Autodesk Inventor part; units mm, degrees
ref_plane "YZ Plane" through (0, 0, 0) normal (1, 0, 0) x (0, 1, 0)
ref_plane "XZ Plane" through (0, 0, 0) normal (0, 1, 0) x (-1, 0, 0)
ref_plane "XY Plane" through (0, 0, 0) normal (0, 0, 1) x (1, 0, 0)
sketch "Sketch1" plane through (0, 0, 0) normal (0, 0, 1) x (1, 0, 0)
  line L0 (0, 0) -> (27.9, 0)
  line L1 (27.9, 0) -> (27.9, -22.1)
  line L2 (27.9, -22.1) -> (0, -22.1)
  line L3 (0, -22.1) -> (0, 0)
  dimension "d0" = 27.9
  dimension "d1" = 22.1
extrude "Extrusion1" add sketch "Sketch1" along normal blind 2.5
sketch "Sketch2" plane through (0, 0, 0) normal (0, 1, 0) x (1, 0, 0)
  line L0 (1.95, -4.5) -> (25.95, -4.5) construction
  line L1 (4.95, -7.5) -> (22.95, -7.5)
  line L2 (22.95, -1.5) -> (4.95, -1.5)
  arc A0 (4.95, -1.5) -> (4.95, -7.5) centre (4.95, -4.5) ccw
  arc A1 (22.95, -7.5) -> (22.95, -1.5) centre (22.95, -4.5) ccw
  line L3 (27.9, 0) -> (27.9, -2.5)
  line L4 (0, 0) -> (0, -2.5)
  line L5 (27.9, -2.5) -> (0, -2.5)
  circle A2 centre (5.95, -4.5) radius 1.6
  circle A3 centre (21.95, -4.5) radius 1.6
  line L6 (4.752, -3.4394) -> (4.752, -5.5606)
  line L7 (0, 0) -> (27.9, 0)
  line L8 (13.95, 0) -> (13.95, -7.0714)
  point P0 (13.95, -4.5)
  dimension "d4" = 6
  dimension "d5" = 24
  dimension "d8" = 1
  dimension "d9" = 3.2
  dimension "d10" = 3.2
  dimension "d11" = 16
  dimension "d12" = 8
extrude "Extrusion2" add sketch "Sketch2" along normal blind 1.5 contours A0 L5 A1 L1 | A0 L2 L8 L5 | L5 L8 L2 A1
fillet "Fillet1" radius 0.3 4 edges at (1.95, 1.5, 4.5) (13.95, 1.5, 7.5) (25.95, 1.5, 4.5) (13.95, 1.5, 1.5)
fillet "Fillet2" radius 0.5 3 edges at (13.95, 0, 1.5) (13.95, 0, 0) (13.95, 0, 2.5)
fillet "Fillet3" radius 0.3 3 edges at (25.5481, 0, 6) (2.3519, 0, 6) (13.95, 0, 7.5)
sketch "Sketch3" plane through (0, 0, 0) normal (0, 0, -1) x (-1, 0, 0)
  circle A0 centre (-24.4, -18.6) radius 2.15
  line L0 (-27.9, -22.1) -> (-27.9, -0.5)
  line L1 (0, -22.1) -> (-27.9, -22.1)
  line L2 (-13.95, -22.1) -> (-13.95, -20.8715)
  circle A1 centre (-24.4, -8.6) radius 2.15
  line L3 (0, 0) -> (-27.9, 0)
  circle A2 centre (-3.5, -18.6) radius 2.15
  circle A3 centre (-3.5, -8.6) radius 2.15
  point P0 (-27.9, -11.3)
  point P1 (0, -11.3)
  dimension "d19" = 4.3
  dimension "d23" = 3.5
  dimension "d28" = 8.6
  dimension "d29" = 3.5
  dimension "d30" = 4.3
  dimension "d31" = 3.5
fillet "Fillet4" radius 0.3 12 edges at (27.9, -0.1464, 0.1464) (27.9, 0, 1.5) (27.9, -11.3, 0) (27.9, -11.05, 2.5) (13.95, -22.1, 0) (27.9, -22.1, 1.25) (13.95, -22.1, 2.5) (0, -22.1, 1.25) (0, -0.1464, 0.1464) (0, 0, 1.5) (0, -11.3, 0) (0, -11.05, 2.5)
extrude "Extrusion3" cut sketch "Sketch3" against normal blind 5
properties part number "distance_sensor_hold"
Geometry check sheet. Reference: the model listing, model coordinates, mm. A direction names the side the tool comes from. Round coordinates to 2 decimals unless told otherwise and drop trailing zeros. Write each loop counter-clockwise with the first axis right and the second up, starting at its lowest first coordinate (ties: lowest second). Pieces come first, ordered by that corner, then holes. Notation, with made-up numbers: (-29.5, 76.5) - (-23.5, 76.5) arc R24 cw to (-23.5, 87.5) - close; hole circle Ø6 at (86, -10). An arc over 180 degrees is marked (long way). One line per item, written item: value.
1. Set-up check for faces 5 (the face through (14, 1.5, 4)), 6 (the face through (14, 0, 5)), 7 (the face through (13.8, 0, 0.8)): record each of +Z, -Z, +X, -X, +Y, -Y from which the full face is reachable in a straight line by a thin tool's end or side.
The answers:
face 5: +Z, -Z, +X, -X, +Y
face 6: +Z, +X, -X, -Y
face 7: -Z, +Y
2. Cross-section at C-C on x = 10.5. Record the boundary of the cut face in (y, z).
The answers:
outline: (-22.1, 0.3) arc R0.3 ccw to (-21.8, 0) - (-0.5, 0) arc R0.5 ccw to (0, 0.5) - (0, 1) arc R0.5 cw to (0.5, 1.5) - (1.2, 1.5) arc R0.3 ccw to (1.5, 1.8) - (1.5, 7.2) arc R0.3 ccw to (1.2, 7.5) - (0.3, 7.5) arc R0.3 ccw to (0, 7.2) - (0, 3) arc R0.5 cw to (-0.5, 2.5) - (-21.8, 2.5) arc R0.3 ccw to (-22.1, 2.2) - close
3. Depth check by flat-ended pin: pin 1 Ø11 at (x, y) = (15, -13.5) entering from +Z; pin 2 Ø4 at (x, y) = (3.5, -18.6) entering from -Z; pin 3 Ø0.6 at (x, z) = (8, 1) entering from +Y; pin 4 Ø4.5 at (x, z) = (18, 6) entering from -Y. Enter the tip coordinate at first touch or a pass-through.
The answers:
pin 1: stops at z = 2.5
pin 2: passes through
pin 3: stops at y = 0.1
pin 4: stops at y = 0
4. Cross-section at B-B on y = -7. Record the boundary of the cut face in (x, z).
The answers:
outline: (0, 0.3) arc R0.3 ccw to (0.3, 0) - (2.06, 0) - (2.06, 2.5) - (0.3, 2.5) arc R0.3 ccw to (0, 2.2) - close; (4.94, 0) - (22.96, 0) - (22.96, 2.5) - (4.94, 2.5) - close; (25.84, 0) - (27.6, 0) arc R0.3 ccw to (27.9, 0.3) - (27.9, 2.2) arc R0.3 ccw to (27.6, 2.5) - (25.84, 2.5) - close
5. Scan lines: L1, parallel to X at y = 0.65, z = 4.5; L2, parallel to Y at x = 3.5, z = 0.6; L3, parallel to Z at x = 21.95, y = 0.7. Record each from-to range of solid material in increasing order.
The answers:
L1: x = 1.95 to 4.35, 7.55 to 20.35, 23.55 to 25.95
L2: y = -22.1 to -20.75, -16.45 to -10.75, -6.45 to 0
L3: z = 1.5 to 2.9, 6.1 to 7.5
6. Mould release check, pull along Z, two halves, no side actions. Record for faces 1 (the face through (6.69, 0.74, 3.08)), 2 (the face through (14, 1, 7.5)), 3 (the face through (23.43, 0.74, 3.89)), 4 (the face through (5.206, -9.908, 1.232)): released by +Z, released by -Z, zero draft, split by the parting line, or undercut.
The answers:
face 1: undercut
face 2: released by +Z
face 3: undercut
face 4: zero draft
7. Cross-section at A-A on z = 4.5. Record the boundary of the cut face in (x, y), and give its area (3 significant figures).
The answers:
outline: (1.95, 0.3) arc R0.3 ccw to (2.25, 0) - (4.35, 0) - (4.35, 1.5) - (2.25, 1.5) arc R0.3 ccw to (1.95, 1.2) - close; (7.55, 0) - (20.35, 0) - (20.35, 1.5) - (7.55, 1.5) - close; (23.55, 0) - (25.65, 0) arc R0.3 ccw to (25.95, 0.3) - (25.95, 1.2) arc R0.3 ccw to (25.65, 1.5) - (23.55, 1.5) - close
area: 26.3 mm^2
